Source: CAD feature listing. Evaluate the final solid. Frame: model axes, mm. Face numbers are marked on the shaded views. Give positions to 0.01 mm unless a question says otherwise; leave off trailing zeros. One line per item, written item: value. Start each with the question number.
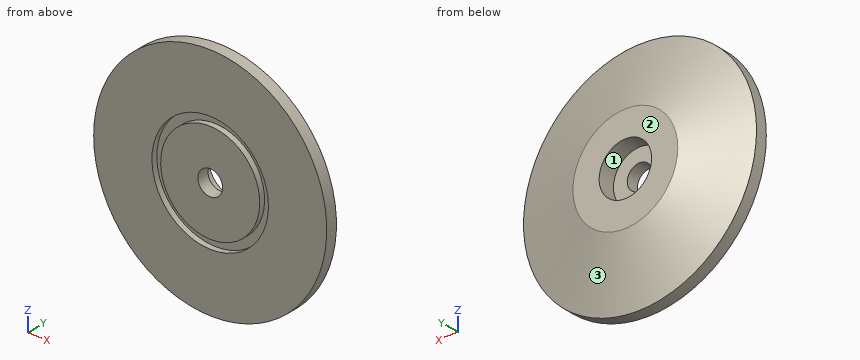
from build123d import *

# Parameters (mm, degrees)
SKETCH2_W                                = 4.7625
SKETCH2_H                                = 3.175
CBORE_FOR_1_2_HEX_HEAD_BOLT1_D           = 13.49248
CBORE_FOR_1_2_HEX_HEAD_BOLT1_CBORE_D     = 28.575
CBORE_FOR_1_2_HEX_HEAD_BOLT1_CBORE_DEPTH = 9.2456


with BuildPart() as part:
    # Sketch1 → Base-Revolve (revolve)
    with BuildSketch(Plane.XY, mode=Mode.PRIVATE) as base_revolve_sk:
        Polygon((0, 0), (63.5, 0), (63.5, 6.35), (28.575, 15.875), (0, 15.875), align=None)
    revolve(base_revolve_sk.sketch.rotate(Axis((0, 15.875, 0), (0, -1, 0)), 180), axis=Axis((0, 15.875, 0), (0, -1, 0)))

    # Sketch2 → Groove (revolve, cut)
    with BuildSketch(Plane.XY, mode=Mode.PRIVATE) as groove_sk:
        with Locations((29.36875, 1.5875)):
            Rectangle(SKETCH2_W, SKETCH2_H)
    revolve(groove_sk.sketch.rotate(Axis((0, 0, 0), (0, 1, 0)), 90), axis=Axis((0, 0, 0), (0, 1, 0)), mode=Mode.SUBTRACT)

    # CBORE for 1/2 Hex Head Bolt1 (through all)
    with Locations(Plane(origin=(0, 15.875, 0), x_dir=(-1, 0, 0), z_dir=(0, 1, 0))):
        with Locations((0, 0)):
            CounterBoreHole(CBORE_FOR_1_2_HEX_HEAD_BOLT1_D / 2, CBORE_FOR_1_2_HEX_HEAD_BOLT1_CBORE_D / 2, CBORE_FOR_1_2_HEX_HEAD_BOLT1_CBORE_DEPTH)


solid = part.part
1. Draft query along Z for the marked faces 1, 2 and 3. Return one class per face: pulls with the +Z half, pulls with the -Z half, needs draft (parallel to the pull), parting line crosses it, or undercut.
2. Ray query, L1, parallel to Z at x = 0, y = 3.25; L2, parallel to Z at x = 1.5, y = 1; L3, parallel to X at y = 1.25, z = 55. Return the intervals inside material, ascending.
3. Contact query for flat-ended pins moving along their axis: pin 1 Ø8 at (x, z) = (-5, -41.5) entering from +Y; pin 2 Ø1 at (y, z) = (4.5, -36) entering from -X; pin 3 Ø6 at (x, y) = (-28, 4) entering from -Z. Output: stop coordinate, or through.
Data:
1. face 1: undercut
1. face 2: needs draft
1. face 3: parting line crosses it
2. L1: z = -63.5 to -6.75, 6.75 to 63.5
2. L2: z = -63.48 to -31.71, -26.95 to -6.58, 6.58 to 26.95, 31.71 to 63.48
2. L3: x = -31.74 to 31.74
3. pin 1: stops at y = 13.36
3. pin 2: stops at x = -52.65
3. pin 3: stops at z = -58.37
